```python
from build123d import *

# Parameters (mm, degrees)
SKIZZE2_W                            = 67.3333
SKIZZE2_H                            = 68
SCHNITT_LINEAR_AUSTRAGEN1_DEPTH      = 30
SCHNITT_LINEAR_AUSTRAGEN1_DEPTH_BACK = 30


with BuildPart() as part:
    # Skizze1 → Rotation1 (revolve)
    with BuildSketch(Plane(origin=(0, 0, 0), x_dir=(0, 0, -1), z_dir=(1, 0, 0))):
        Polygon((0, 4.1), (0.5, 3.6), (2, 3.6), (2, 4.9), (10.8, 4.9), (10.8, 4.4585), (13.9585, 4.4585), (14.5, 5), (14.5, 6.5), (14.299038106, 7.25), (1.25, 7.25), (0, 6), align=None)
    revolve(axis=Axis((0, 0, -14.5), (0, 0, 1)))

    # Skizze2 → Schnitt-Linear austragen1 (cut, two sides)
    with BuildSketch(Plane.XY) as schnitt_linear_austragen1_sk:
        with Locations((-1.08335, 0.1667)):
            Rectangle(SKIZZE2_W, SKIZZE2_H)
        Polygon((-6.5, -3.75277675), (0, -7.505553499), (6.5, -3.75277675), (6.5, 3.75277675), (0, 7.505553499), (-6.5, 3.75277675), align=None, mode=Mode.SUBTRACT)
    extrude(amount=SCHNITT_LINEAR_AUSTRAGEN1_DEPTH, mode=Mode.SUBTRACT)
    extrude(schnitt_linear_austragen1_sk.sketch, amount=-SCHNITT_LINEAR_AUSTRAGEN1_DEPTH_BACK, mode=Mode.SUBTRACT)


solid = part.part
```
Can you work these out from the model? Positions are in its coordinate system, mm. A direction names the side the tool comes from. Coordinates: 2 decimals unless noted, no trailing zeros. Write each loop counter-clockwise with the first axis right and the second up, starting at its lowest first coordinate (ties: lowest second). Pieces come first, ordered by that corner, then holes. Notation, with made-up numbers: (9.25, 12) - (14.25, 12) arc R34 cw to (14.25, 48) - close; hole circle Ø7 at (65, 17). An arc over 180 degrees is marked (long way). Return JSON: item names as keys, results as strings.
Q1. On a 3-axis mill with a long thin cutter (end or side, diameter ignored), from which of +Z, -Z, +X, -X, +Y, -Y can I reach the whole of each face in a straight line? I mean faces 4 (the cylindrical face through (2.71, -3.54, -12.4)), 5 (the conical face through (5.839, 3.314, -14.443)). Say none if no direction works.
Computed values:
{"face 4": "-Z", "face 5": "-Z, +X, +Y"}
Q2. If we section it at B-B (z = -11.5): Please give me the cut outline in (x, y).
Computed values:
{"outline": "(-6.5, -3.21) arc R7.25 ccw to (-6.03, -4.02) - (-0.47, -7.23) arc R7.25 ccw to (0.47, -7.23) - (6.03, -4.02) arc R7.25 ccw to (6.5, -3.21) - (6.5, 3.21) arc R7.25 ccw to (6.03, 4.02) - (0.47, 7.23) arc R7.25 ccw to (-0.47, 7.23) - (-6.03, 4.02) arc R7.25 ccw to (-6.5, 3.21) - close; hole circle Ø8.92 at (0, 0)"}
Q3. If we section it at C-C (z = -3): Please give me the cut outline in (x, y), then the cut area to 3 significant figures.
Computed values:
{"outline": "(-6.5, -3.21) arc R7.25 ccw to (-6.03, -4.02) - (-0.47, -7.23) arc R7.25 ccw to (0.47, -7.23) - (6.03, -4.02) arc R7.25 ccw to (6.5, -3.21) - (6.5, 3.21) arc R7.25 ccw to (6.03, 4.02) - (0.47, 7.23) arc R7.25 ccw to (-0.47, 7.23) - (-6.03, 4.02) arc R7.25 ccw to (-6.5, 3.21) - close; hole circle Ø9.8 at (0, 0)", "area": "70.2 mm2"}
Q4. Thinking about a two-plate mould opening in Z: for faces 1 (the flat face through (5, -2, -14.5)), 2 (the flat face through (6.5, 0, -7)), 3 (the cylindrical face through (4.783, -1.062, -6.462)), which applies, +Z half, -Z half, draft (parallel to the pull), parting line (faces both ways), or undercut?
Computed values:
{"face 1": "-Z half", "face 2": "draft", "face 3": "undercut"}
Q5. If we section it at A-A (x = 0): Please give me the cut outline in (y, z), then the cut area to 3 significant figures.
Computed values:
{"outline": "(-7.25, -14.3) - (-6.5, -14.5) - (-5, -14.5) - (-4.46, -13.96) - (-4.46, -10.8) - (-4.9, -10.8) - (-4.9, -2) - (-3.6, -2) - (-3.6, -0.5) - (-4.1, 0) - (-6, 0) - (-7.25, -1.25) - close; (3.6, -2) - (4.9, -2) - (4.9, -10.8) - (4.46, -10.8) - (4.46, -13.96) - (5, -14.5) - (6.5, -14.5) - (7.25, -14.3) - (7.25, -1.25) - (6, 0) - (4.1, 0) - (3.6, -0.5) - close", "area": "74.4 mm2"}
Q6. I'm going to push flat-ended pins straight in: pin 1 Ø4 at (x, z) = (4, -5.5) entering from -Y; pin 2 Ø4 at (y, z) = (4.5, -6.5) entering from +X; pin 3 Ø5 at (x, z) = (-3, -11.5) entering from -Y. Where does each tip first touch, or does it pass through?
Computed values:
{"pin 1": "stops at y = -6.35", "pin 2": "stops at x = 6.5", "pin 3": "stops at y = -7.22"}
Q7. Please list where these lines run through material, in increasing order: L1, parallel to X at y = 0, z = -0.9; L2, parallel to Y at x = 0, z = -11.9; L3, parallel to X at y = 0, z = -7.5. Write a range as from..to.
Computed values:
{"L1": "x = -6.5..-3.6, 3.6..6.5", "L2": "y = -7.25..-4.46, 4.46..7.25", "L3": "x = -6.5..-4.9, 4.9..6.5"}
